Could you check a few things on this model? Use its own coordinates, in mm. Face numbers are marked on the shaded views. A direction names the side the tool comes from. Coordinates: 2 decimals unless noted, no trailing zeros. Loops run counter-clockwise (first coordinate to the right, second up) from the corner with the lowest first, then second, coordinate; pieces in that order, holes last. Notation, with made-up numbers: (86.25, 43) - (125.25, 43) arc R23 cw to (125.25, 79) - close; hole circle Ø1 at (-2, 11.25). An arc over 180 degrees is marked (long way). One line per item, written item: value. Start each with the question number.
(1) If we section it at B-B on z = 9.5: Write out the boundary of the cut face in (x, y).
(2) If we section it at C-C on y = 21.5: Write out the boundary of the cut face in (x, z).
(3) If we section it at A-A on x = -10: Write out the boundary of the cut face in (y, z), then the cut area to 3 significant figures.
(4) If we mould it in two halves opening along Y, with no side actions, what happens to the marked faces 3, 4 and 5? For each: pulls with the +Y half, pulls with the -Y half, needs draft (parallel to the pull), parting line crosses it, or undercut.
(5) I'm going to push a flat-ended pin straight in: P1, Ø2, axis at x = -15.5, y = 9, coming from the +Z side. Where does the tip first touch, or does it pass through?
(6) If I drill on line 1 along Y through (x, z) = (-24.5, 8.5); line 2 along X through (y, z) = (24.5, 21); line 3 along Z through (x, y) = (10, 22), over which ranges is the centre line in solid material (lowest first)? Write a range as from..to.
(7) On a 3-axis mill with a long thin cutter (end or side, diameter ignored), from which of +Z, -Z, +X, -X, +Y, -Y can I reach the whole of each face in a straight line? I mean the marked faces 1 and 2. Say none if no direction works.
(8) If we section it at D-D on x = 24: Write out the boundary of the cut face in (y, z).
```python
from build123d import *

# Parameters (mm, degrees)
F0_W     = 80
F0_H     = 54
F1_DEPTH = 7
F3_DEPTH = 7
F5_R     = 3.5
F6_DEPTH = 54.001


with BuildPart() as f1:
    # F0 (on Top) → F1 (new body)
    with BuildSketch(Plane.XY):
        Rectangle(F0_W, F0_H)
    extrude(amount=F1_DEPTH)

    # F2 (on face) → F3 (join)
    with BuildSketch(Plane.XZ.offset(27)):
        with BuildLine():
            Line((17.5, 30.876799), (-17.5, 30.876799))
            ThreePointArc((-17.5, 30.876799), (-24.137327, 14.591705), (-40, 7))
            Line((-40, 7), (40, 7))
            ThreePointArc((40, 7), (24.137307, 14.591686), (17.5, 30.876799))
        make_face()
    extrude(amount=-F3_DEPTH)

    # F4: F1 across plane


with BuildPart() as f1_1:
    add(f1.part)
    add(f1.part.mirror(Plane.XZ))

    # F5 (on face) → F6 (cut, through all)
    with BuildSketch(Plane.XZ.offset(27)):
        with Locations((-10, 20.678958)):
            Circle(F5_R)
        with Locations((10, 20.678958)):
            Circle(F5_R)
    extrude(amount=-F6_DEPTH, mode=Mode.SUBTRACT)


solid = f1_1.part
```
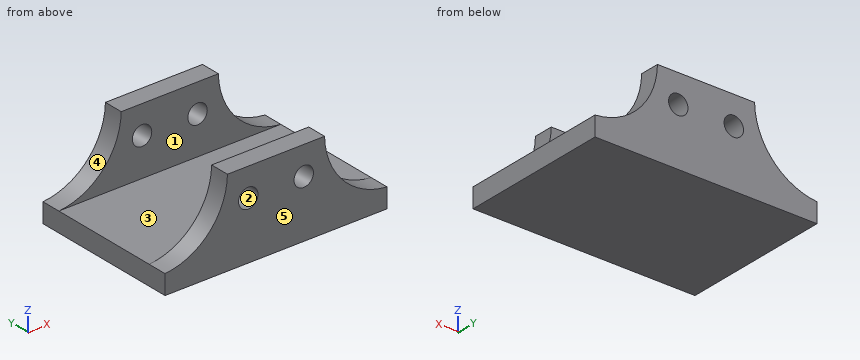
Values:
1. outline: (-30.99, -27) - (30.99, -27) - (30.99, -20) - (-30.99, -20) - close; (-30.99, 20) - (30.99, 20) - (30.99, 27) - (-30.99, 27) - close
2. outline: (-40, 0) - (40, 0) - (40, 7) arc R24.4 cw to (17.5, 30.88) - (-17.5, 30.88) arc R24.4 cw to (-40, 7) - close; hole circle Ø7 at (-10, 20.68); hole circle Ø7 at (10, 20.68)
3. outline: (-27, 0) - (27, 0) - (27, 17.18) - (20, 17.18) - (20, 7) - (-20, 7) - (-20, 17.18) - (-27, 17.18) - close; (-27, 24.18) - (-20, 24.18) - (-20, 30.88) - (-27, 30.88) - close; (20, 24.18) - (27, 24.18) - (27, 30.88) - (20, 30.88) - close
3. area: 614 mm2
4. face 3: undercut
4. face 4: needs draft
4. face 5: pulls with the -Y half
5. P1: stops at z = 7
6. line 1: y = -27..-20, 20..27
6. line 2: x = -19.79..-13.49, -6.51..6.51, 13.49..19.79
6. line 3: z = 0..17.18, 24.18..30.88
7. face 1: +Z, +X, -X
7. face 2: +Y, -Y
8. outline: (-27, 0) - (27, 0) - (27, 14.74) - (20, 14.74) - (20, 7) - (-20, 7) - (-20, 14.74) - (-27, 14.74) - close
